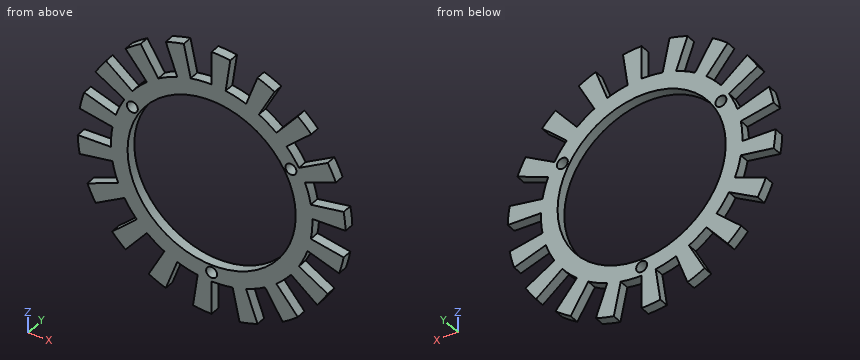
from build123d import *

# Parameters (mm, degrees)
SKETCH1_R           = 30.25
SKETCH1_R_2         = 25.25
EXTRUDE_THIN1_DEPTH = 3
SKETCH2_R           = 1.65
CUT_EXTRUDE3_DEPTH  = 10
BOSS_EXTRUDE1_DEPTH = 3


with BuildPart() as part:
    # Sketch1 → Extrude-Thin1 (new body)
    with BuildSketch(Plane(origin=(0, 0, 0), x_dir=(1, 0, 0), z_dir=(0, 1, 0))):
        Circle(SKETCH1_R)
        Circle(SKETCH1_R_2, mode=Mode.SUBTRACT)
    extrude(amount=-EXTRUDE_THIN1_DEPTH)

    # Sketch2 → Cut-Extrude3 (cut)
    with BuildSketch(Plane(origin=(0, 0, 0), x_dir=(1, 0, 0), z_dir=(0, 1, 0))):
        with Locations((0, 27.5)):
            Circle(SKETCH2_R)
        with Locations((23.815698604, -13.75)):
            Circle(SKETCH2_R)
        with Locations((-23.815698604, -13.75)):
            Circle(SKETCH2_R)
    extrude(amount=-CUT_EXTRUDE3_DEPTH, mode=Mode.SUBTRACT)

    # Sketch5 → Boss-Extrude1 (add)
    with BuildSketch(Plane.XZ.offset(3)):
        with BuildLine():
            Line((0, 40.25), (0, 30.25))
            ThreePointArc((0, 30.25), (2.110133331, 30.17631252), (4.209986304, 29.955609079))
            Line((4.209986304, 29.955609079), (5.601717314, 39.858289767))
            ThreePointArc((5.601717314, 39.858289767), (2.807698068, 40.151953023), (0, 40.25))
        make_face()
        with BuildLine():
            Line((13.766310769, 37.822627987), (10.346109336, 28.425701779))
            ThreePointArc((10.346109336, 28.425701779), (12.303783453, 27.634750094), (14.201514774, 26.709164684))
            Line((14.201514774, 26.709164684), (18.896230402, 35.538640613))
            ThreePointArc((18.896230402, 35.538640613), (16.371149884, 36.77020467), (13.766310769, 37.822627987))
        make_face()
        with BuildLine():
            Line((25.87220129, 30.833288836), (19.444325193, 23.172844404))
            ThreePointArc((19.444325193, 23.172844404), (21.013415706, 21.76002896), (22.480130971, 20.241200842))
            Line((22.480130971, 20.241200842), (29.911579225, 26.932506906))
            ThreePointArc((29.911579225, 26.932506906), (27.959999411, 28.953426964), (25.87220129, 30.833288836))
        make_face()
        with BuildLine():
            Line((34.857522502, 20.125), (26.197268464, 15.125))
            ThreePointArc((26.197268464, 15.125), (27.188519901, 13.26072719), (28.047311601, 11.331849451))
            Line((28.047311601, 11.331849451), (37.319150146, 15.077915385))
            ThreePointArc((37.319150146, 15.077915385), (36.176460364, 17.644438658), (34.857522502, 20.125))
        make_face()
        with BuildLine():
            Line((39.638512059, 6.989339151), (29.790434529, 5.252857374))
            ThreePointArc((29.790434529, 5.252857374), (30.084287335, 3.161986014), (30.231572517, 1.055709775))
            Line((30.231572517, 1.055709775), (40.225480788, 1.404704742))
            ThreePointArc((40.225480788, 1.404704742), (40.029506289, 4.207270647), (39.638512059, 6.989339151))
        make_face()
        with BuildLine():
            Line((39.638512059, -6.989339151), (29.790434529, -5.252857374))
            ThreePointArc((29.790434529, -5.252857374), (29.35144572, -7.318137342), (28.769459618, -9.34776408))
            Line((28.769459618, -9.34776408), (38.280024781, -12.437934024))
            ThreePointArc((38.280024781, -12.437934024), (39.054402983, -9.737356298), (39.638512059, -6.989339151))
        make_face()
        with BuildLine():
            Line((34.857522502, -20.125), (26.197268464, -15.125))
            ThreePointArc((26.197268464, -15.125), (25.07838657, -16.91558533), (23.837325297, -18.623759629))
            Line((23.837325297, -18.623759629), (31.717432833, -24.780374382))
            ThreePointArc((31.717432833, -24.780374382), (33.368762295, -22.507514365), (34.857522502, -20.125))
        make_face()
        with BuildLine():
            Line((25.87220129, -30.833288836), (19.444325193, -23.172844404))
            ThreePointArc((19.444325193, -23.172844404), (17.780503882, -24.47276408), (16.030057743, -25.653454909))
            Line((16.030057743, -25.653454909), (21.329250385, -34.13393587))
            ThreePointArc((21.329250385, -34.13393587), (23.658356405, -32.562934024), (25.87220129, -30.833288836))
        make_face()
        with BuildLine():
            Line((13.766310769, -37.822627987), (10.346109336, -28.425701779))
            ThreePointArc((10.346109336, -28.425701779), (8.338030013, -29.078166302), (6.289328647, -29.588964922))
            Line((6.289328647, -29.588964922), (8.368445555, -39.37044093))
            ThreePointArc((8.368445555, -39.37044093), (11.094403572, -38.690783262), (13.766310769, -37.822627987))
        make_face()
        with BuildLine():
            Line((0, -40.25), (0, -30.25))
            ThreePointArc((0, -30.25), (-2.110133331, -30.17631252), (-4.209986304, -29.955609079))
            Line((-4.209986304, -29.955609079), (-5.601717314, -39.858289767))
            ThreePointArc((-5.601717314, -39.858289767), (-2.807698068, -40.151953023), (0, -40.25))
        make_face()
        with BuildLine():
            Line((-13.766310769, -37.822627987), (-10.346109336, -28.425701779))
            ThreePointArc((-10.346109336, -28.425701779), (-12.303783453, -27.634750094), (-14.201514774, -26.709164684))
            Line((-14.201514774, -26.709164684), (-18.896230402, -35.538640613))
            ThreePointArc((-18.896230402, -35.538640613), (-16.371149884, -36.77020467), (-13.766310769, -37.822627987))
        make_face()
        with BuildLine():
            Line((-25.87220129, -30.833288836), (-19.444325193, -23.172844404))
            ThreePointArc((-19.444325193, -23.172844404), (-21.013415706, -21.76002896), (-22.480130971, -20.241200842))
            Line((-22.480130971, -20.241200842), (-29.911579225, -26.932506906))
            ThreePointArc((-29.911579225, -26.932506906), (-27.959999411, -28.953426964), (-25.87220129, -30.833288836))
        make_face()
        with BuildLine():
            Line((-34.857522502, -20.125), (-26.197268464, -15.125))
            ThreePointArc((-26.197268464, -15.125), (-27.188519901, -13.26072719), (-28.047311601, -11.331849451))
            Line((-28.047311601, -11.331849451), (-37.319150146, -15.077915385))
            ThreePointArc((-37.319150146, -15.077915385), (-36.176460364, -17.644438658), (-34.857522502, -20.125))
        make_face()
        with BuildLine():
            Line((-39.638512059, -6.989339151), (-29.790434529, -5.252857374))
            ThreePointArc((-29.790434529, -5.252857374), (-30.084287335, -3.161986014), (-30.231572517, -1.055709775))
            Line((-30.231572517, -1.055709775), (-40.225480788, -1.404704742))
            ThreePointArc((-40.225480788, -1.404704742), (-40.029506289, -4.207270647), (-39.638512059, -6.989339151))
        make_face()
        with BuildLine():
            Line((-39.638512059, 6.989339151), (-29.790434529, 5.252857374))
            ThreePointArc((-29.790434529, 5.252857374), (-29.35144572, 7.318137342), (-28.769459618, 9.34776408))
            Line((-28.769459618, 9.34776408), (-38.280024781, 12.437934024))
            ThreePointArc((-38.280024781, 12.437934024), (-39.054402983, 9.737356298), (-39.638512059, 6.989339151))
        make_face()
        with BuildLine():
            Line((-34.857522502, 20.125), (-26.197268464, 15.125))
            ThreePointArc((-26.197268464, 15.125), (-25.07838657, 16.91558533), (-23.837325297, 18.623759629))
            Line((-23.837325297, 18.623759629), (-31.717432833, 24.780374382))
            ThreePointArc((-31.717432833, 24.780374382), (-33.368762295, 22.507514365), (-34.857522502, 20.125))
        make_face()
        with BuildLine():
            Line((-25.87220129, 30.833288836), (-19.444325193, 23.172844404))
            ThreePointArc((-19.444325193, 23.172844404), (-17.780503882, 24.47276408), (-16.030057743, 25.653454909))
            Line((-16.030057743, 25.653454909), (-21.329250385, 34.13393587))
            ThreePointArc((-21.329250385, 34.13393587), (-23.658356405, 32.562934024), (-25.87220129, 30.833288836))
        make_face()
        with BuildLine():
            Line((-13.766310769, 37.822627987), (-10.346109336, 28.425701779))
            ThreePointArc((-10.346109336, 28.425701779), (-8.338030013, 29.078166302), (-6.289328647, 29.588964922))
            Line((-6.289328647, 29.588964922), (-8.368445555, 39.37044093))
            ThreePointArc((-8.368445555, 39.37044093), (-11.094403572, 38.690783262), (-13.766310769, 37.822627987))
        make_face()
    extrude(amount=-BOSS_EXTRUDE1_DEPTH)


solid = part.part
The model under review builds one solid part; all positions refer to its coordinate system, in mm. Coordinates: 2 decimals unless noted, no trailing zeros. Loops run counter-clockwise (first coordinate to the right, second up) from the corner with the lowest first, then second, coordinate; pieces in that order, holes last. Notation, with made-up numbers: M 75,74.25 L 83,74.25 A25 cw 83,112.25 Z; hole C 69,6.5 d11. An arc over 180 degrees is marked long. Put each result on its own line as item: value. Start each with the question number.
Q1. Wall thickness on line 1 (Z direction, x = -35, y = -0.95); line 2 (Z direction, x = -32.5, y = -0.85); line 3 (X direction, y = -0.8, z = 13.75): over which ranges is each line inside the solid? List them lowest first.
Q2. Add section B-B (z = 13.75). Write out the cut boundary in (x, y).
Q3. Clearance check with a flat-ended pin moving along its axis: pin 1 (0.9 mm diameter, centred on y = -1, z = -33.5, fed in from +X). State where the tip first meets the part, or that it passes through.
Q4. Add section C-C (y = -2.3). Count the separate pieces of the cut face and the enclosed holes in it, and give its area (3 significant figures).
Q5. Add section A-A (z = 0). Write out the cut boundary in (x, y), and give its area (3 significant figures).
Answers:
1. line 1: z = -19.88 to -14.14, -6.17 to -1.22, 6.17 to 11.37
1. line 2: z = -18.76 to -13.13, -5.73 to -1.13, 5.73 to 10.56, 18.76 to 23.74
1. line 3: x = -26.94 to -25.47, -22.17 to -21.18, 21.18 to 22.17, 25.47 to 34.03
2. outline: M -26.94,-3 L -25.47,-3 L -25.47,0 L -26.94,0 Z; M -22.17,-3 L -21.18,-3 L -21.18,0 L -22.17,0 Z; M 21.18,-3 L 22.17,-3 L 22.17,0 L 21.18,0 Z; M 25.47,-3 L 34.03,-3 L 34.03,0 L 25.47,0 Z
3. pin 1: stops at x = 22.97
4. separate pieces: 1
4. enclosed holes: 4
4. area: 1,730 mm^2
5. outline: M -30.25,-3 L -25.25,-3 L -25.25,0 L -30.25,0 Z; M 25.25,-3 L 30.25,-3 L 30.25,0 L 25.25,0 Z
5. area: 30.0 mm^2
